```python
from build123d import *

# Parameters (mm, degrees)
SKETCH1_R           = 76.2
BOSS_EXTRUDE1_DEPTH = 6.35
SKETCH2_R           = 35
CUT_EXTRUDE1_DEPTH  = 6.35
SKETCH3_R           = 6.35
CUT_EXTRUDE2_DEPTH  = 10
SKETCH7_R           = 1.5875
CUT_EXTRUDE4_DEPTH  = 10
SKETCH8_R           = 6.35
CUT_EXTRUDE5_DEPTH  = 10
SKETCH9_R           = 38.1
CUT_EXTRUDE6_DEPTH  = 10
CUT_EXTRUDE10_DEPTH = 10


with BuildPart() as part:
    # Sketch1 → Boss-Extrude1 (new body)
    with BuildSketch(Plane(origin=(0, 0, 0), x_dir=(1, 0, 0), z_dir=(0, 1, 0))):
        with Locations(Location((0, 0, 0), (0, 0, 270))):
            Circle(SKETCH1_R)
    extrude(amount=BOSS_EXTRUDE1_DEPTH)

    # Sketch2 → Cut-Extrude1 (cut)
    with BuildSketch(Plane(origin=(0, 6.35, 0), x_dir=(1, 0, 0), z_dir=(0, 1, 0))):
        with Locations(Location((0, 0, 0), (0, 0, 270))):
            Circle(SKETCH2_R)
    extrude(amount=-CUT_EXTRUDE1_DEPTH, mode=Mode.SUBTRACT)

    # Sketch3 → Cut-Extrude2 (cut)
    with BuildSketch(Plane(origin=(0, 6.35, 0), x_dir=(1, 0, 0), z_dir=(0, 1, 0))):
        with Locations(Location((-64.2875, 0, 0), (0, 0, 270))):
            Circle(SKETCH3_R)
        with Locations(Location((64.2875, 0, 0), (0, 0, 270))):
            Circle(SKETCH3_R)
    extrude(amount=-CUT_EXTRUDE2_DEPTH, mode=Mode.SUBTRACT)

    # Sketch7 → Cut-Extrude4 (cut)
    with BuildSketch(Plane(origin=(0, 6.35, 0), x_dir=(1, 0, 0), z_dir=(0, 1, 0))):
        with Locations(Location((-24.5999, 59.5249, 0), (0, 0, 270))):
            Circle(SKETCH7_R)
        with Locations(Location((24.5999, 59.5249, 0), (0, 0, 270))):
            Circle(SKETCH7_R)
        with Locations(Location((24.5999, -59.5249, 0), (0, 0, 270))):
            Circle(SKETCH7_R)
        with Locations(Location((-24.5999, -59.5249, 0), (0, 0, 270))):
            Circle(SKETCH7_R)
        with Locations(Location((-59.5249, 24.5999, 0), (0, 0, 270))):
            Circle(SKETCH7_R)
        with Locations(Location((-59.5249, -24.5999, 0), (0, 0, 270))):
            Circle(SKETCH7_R)
        with Locations(Location((59.5249, 24.5999, 0), (0, 0, 270))):
            Circle(SKETCH7_R)
        with Locations(Location((59.5249, -24.5999, 0), (0, 0, 270))):
            Circle(SKETCH7_R)
    extrude(amount=-CUT_EXTRUDE4_DEPTH, mode=Mode.SUBTRACT)

    # Sketch8 → Cut-Extrude5 (cut)
    with BuildSketch(Plane(origin=(0, 6.35, 0), x_dir=(1, 0, 0), z_dir=(0, 1, 0))):
        with Locations(Location((-64.2875, 0, 0), (0, 0, 270))):
            Circle(SKETCH8_R)
        with Locations(Location((64.2875, 0, 0), (0, 0, 270))):
            Circle(SKETCH8_R)
        with Locations(Location((0, -64.2875, 0), (0, 0, 270))):
            Circle(SKETCH8_R)
        with Locations(Location((0, 64.2875, 0), (0, 0, 270))):
            Circle(SKETCH8_R)
    extrude(amount=-CUT_EXTRUDE5_DEPTH, mode=Mode.SUBTRACT)

    # Sketch9 → Cut-Extrude6 (cut)
    with BuildSketch(Plane(origin=(0, 6.35, 0), x_dir=(1, 0, 0), z_dir=(0, 1, 0))):
        with Locations(Location((0, 0, 0), (0, 0, 270))):
            Circle(SKETCH9_R)
    extrude(amount=-CUT_EXTRUDE6_DEPTH, mode=Mode.SUBTRACT)

    # Sketch10 → Cut-Extrude10 (cut)
    with BuildSketch(Plane(origin=(0, 6.35, 0), x_dir=(1, 0, 0), z_dir=(0, 1, 0))):
        with BuildLine():
            Line((-22.744667262, 45.067306456), (-25.69340518, 50.731779293))
            ThreePointArc((-25.69340518, 50.731779293), (-29.722021798, 53.943778286), (-34.806582189, 53.110750666))
            ThreePointArc((-34.806582189, 53.110750666), (-44.649726855, 45.151432888), (-52.718528787, 35.397834998))
            ThreePointArc((-52.718528787, 35.397834998), (-53.599643338, 30.28850003), (-50.378779602, 26.225532708))
            Line((-50.378779602, 26.225532708), (-44.706731925, 23.272851578))
            ThreePointArc((-44.706731925, 23.272851578), (-40.248145008, 22.741576978), (-36.552799702, 25.292199073))
            ThreePointArc((-36.552799702, 25.292199073), (-31.232430693, 31.628116811), (-24.830037796, 36.868302416))
            ThreePointArc((-24.830037796, 36.868302416), (-22.223123282, 40.56995153), (-22.744667262, 45.067306456))
        make_face()
        with BuildLine():
            ThreePointArc((24.830037796, 36.868302416), (22.223123282, 40.56995153), (22.744667262, 45.067306456))
            Line((22.744667262, 45.067306456), (25.69340518, 50.731779293))
            ThreePointArc((25.69340518, 50.731779293), (29.722021798, 53.943778286), (34.806582189, 53.110750666))
            ThreePointArc((34.806582189, 53.110750666), (44.649726855, 45.151432888), (52.718528787, 35.397834998))
            ThreePointArc((52.718528787, 35.397834998), (53.599643338, 30.28850003), (50.378779602, 26.225532708))
            Line((50.378779602, 26.225532708), (44.706731925, 23.272851578))
            ThreePointArc((44.706731925, 23.272851578), (40.248145008, 22.741576978), (36.552799702, 25.292199073))
            ThreePointArc((36.552799702, 25.292199073), (31.232430693, 31.628116811), (24.830037796, 36.868302416))
        make_face()
        with BuildLine():
            Line((22.744667262, -45.067306456), (25.69340518, -50.731779293))
            ThreePointArc((25.69340518, -50.731779293), (29.722021798, -53.943778286), (34.806582189, -53.110750666))
            ThreePointArc((34.806582189, -53.110750666), (44.649726855, -45.151432888), (52.718528787, -35.397834998))
            ThreePointArc((52.718528787, -35.397834998), (53.599643338, -30.28850003), (50.378779602, -26.225532708))
            Line((50.378779602, -26.225532708), (44.706731925, -23.272851578))
            ThreePointArc((44.706731925, -23.272851578), (40.248145008, -22.741576978), (36.552799702, -25.292199073))
            ThreePointArc((36.552799702, -25.292199073), (31.232430693, -31.628116811), (24.830037796, -36.868302416))
            ThreePointArc((24.830037796, -36.868302416), (22.223123282, -40.56995153), (22.744667262, -45.067306456))
        make_face()
        with BuildLine():
            ThreePointArc((-24.830037796, -36.868302416), (-22.223123282, -40.56995153), (-22.744667262, -45.067306456))
            Line((-22.744667262, -45.067306456), (-25.69340518, -50.731779293))
            ThreePointArc((-25.69340518, -50.731779293), (-29.722021798, -53.943778286), (-34.806582189, -53.110750666))
            ThreePointArc((-34.806582189, -53.110750666), (-44.649726855, -45.151432888), (-52.718528787, -35.397834998))
            ThreePointArc((-52.718528787, -35.397834998), (-53.599643338, -30.28850003), (-50.378779602, -26.225532708))
            Line((-50.378779602, -26.225532708), (-44.706731925, -23.272851578))
            ThreePointArc((-44.706731925, -23.272851578), (-40.248145008, -22.741576978), (-36.552799702, -25.292199073))
            ThreePointArc((-36.552799702, -25.292199073), (-31.232430693, -31.628116811), (-24.830037796, -36.868302416))
        make_face()
    extrude(amount=-CUT_EXTRUDE10_DEPTH, mode=Mode.SUBTRACT)


solid = part.part
```
Verification items for the finished model (mm, model axes). Round coordinates to 2 decimals unless told otherwise and drop trailing zeros. Write each loop counter-clockwise with the first axis right and the second up, starting at its lowest first coordinate (ties: lowest second). Pieces come first, ordered by that corner, then holes. Notation, with made-up numbers: (-22.5, -15.5) - (-11.5, -15.5) arc R22 ccw to (-11.5, -3.5) - close; hole circle Ø2 at (-4.5, 59). An arc over 180 degrees is marked (long way). Answer as a JSON object with one key per item and string values. Group by question number.
Q1. Section check D-D, the plane x = -56. Enter the section's corners in (y, z), plus the area to 3 significant figures.
Q2. Go/stop test with flat-tipped pins: pin 1 Ø1.5 at (y, z) = (4.5, 45.5) entering from -X; pin 2 Ø3 at (x, z) = (-24.6, -59.52) entering from -Y; pin 3 Ø1 at (y, z) = (2.5, -59) entering from -X; pin 4 Ø2 at (x, y) = (-44.5, 2) entering from -Z. Record where each tip stops, or that it passes through.
Q3. Thickness scan on line 1 (X direction, y = 4.75, z = 0); line 2 (Z direction, x = -58.5, y = 5); line 3 (Z direction, x = -30, y = 4.75). Record the ranges inside material, lowest first.
Q4. Section check A-A, the plane x = 0. Enter the section's corners in (y, z).
Q5. Section check B-B, the plane z = 0. Enter the section's corners in (x, y), plus the area to 3 significant figures.
Q6. Mould release check, pull along X, two halves, no side actions. Record for faces 1 (the cylindrical face through (-23.183, 3.219, -30.235)), 2 (the cylindrical face through (-46.367, 3.131, -60.47)), 3 (the cylindrical face through (-22.24, 3.22, -40.51)): released by +X, released by -X, zero draft, split by the parting line, or undercut.
Q7. Section check C-C, the plane z = 42. Enter the section's corners in (x, y).
Found:
{
 "1": {"outline": "(0, -51.68) - (6.35, -51.68) - (6.35, 51.68) - (0, 51.68) - close", "area": "656 mm^2"},
 "2": {"pin 1": "stops at x = -61.68", "pin 2": "passes through", "pin 3": "stops at x = -48.83", "pin 4": "stops at z = -62.56"},
 "3": {"line 1": "x = -76.2 to -70.64, -57.94 to -38.1, 38.1 to 57.94, 70.64 to 76.2", "line 2": "z = -48.83 to -25.81, -23.39 to -2.61, 2.61 to 23.39, 25.81 to 48.83", "line 3": "z = -70.05 to -54.01, -32.8 to -23.49, 23.49 to 32.8, 54.01 to 70.05"},
 "4": {"outline": "(0, -76.2) - (6.35, -76.2) - (6.35, -70.64) - (0, -70.64) - close; (0, -57.94) - (6.35, -57.94) - (6.35, -38.1) - (0, -38.1) - close; (0, 38.1) - (6.35, 38.1) - (6.35, 57.94) - (0, 57.94) - close; (0, 70.64) - (6.35, 70.64) - (6.35, 76.2) - (0, 76.2) - close"},
 "5": {"outline": "(-76.2, 0) - (-70.64, 0) - (-70.64, 6.35) - (-76.2, 6.35) - close; (-57.94, 0) - (-38.1, 0) - (-38.1, 6.35) - (-57.94, 6.35) - close; (38.1, 0) - (57.94, 0) - (57.94, 6.35) - (38.1, 6.35) - close; (70.64, 0) - (76.2, 0) - (76.2, 6.35) - (70.64, 6.35) - close", "area": "323 mm^2"},
 "6": {"face 1": "undercut", "face 2": "split by the parting line", "face 3": "undercut"},
 "7": {"outline": "(-63.58, 0) - (-47.63, 0) - (-47.63, 6.35) - (-63.58, 6.35) - close; (-22.03, 0) - (22.03, 0) - (22.03, 6.35) - (-22.03, 6.35) - close; (47.63, 0) - (63.58, 0) - (63.58, 6.35) - (47.63, 6.35) - close"}
}
